Job drawing, mm, ordinate dimensions from the low corner. One solid piece. A direction names the side the tool comes from. Give positions to 0.01 mm unless a question says otherwise; leave off trailing zeros. Order: outer loops, then holes, each group sorted by start corner. A loop starts at its lowest first (then second) coordinate and runs counter-clockwise, first axis right, second up.
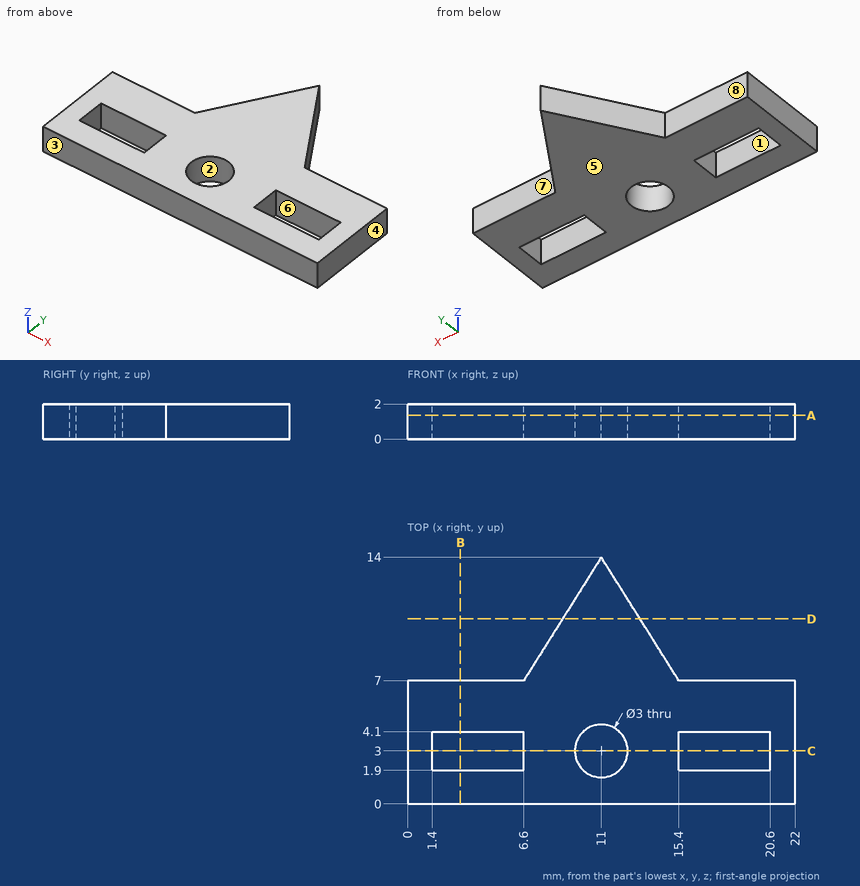
Item 1: Drill centre lines: probe 1 along X at (y, z) = (3.5, 1.85); probe 2 along Y at (x, z) = (16, 0.75); probe 3 along X at (y, z) = (2.75, 0.3). Where is each one in solid material? Low to high.
Item 2: Which spindle directions (+Z, -Z, +X, -X, +Y, -Y) get a long thin tool onto all of the face, cutting with end or side? Do the marked faces 5, 6, 7 and 8. Say none if no direction does.
Item 3: Band-saw the part on C-C on y = 3. List the corners of the cut face in (x, z), plus the area to 3 significant figures.
Item 4: Band-saw the part on D-D on y = 10.5. List the corners of the cut face in (x, z), plus the area to 3 significant figures.
Item 5: Band-saw the part on B-B on x = 3. List the corners of the cut face in (y, z), plus the area to 3 significant figures.
Item 6: Drop a flat-ended pin along its axis: P1, Ø0.6, axis at x = 2.5, z = 0.5, coming from the +Y side. Give the stop position or say it passes through.
Item 7: Band-saw the part on A-A on z = 1.35. List the corners of the cut face in (x, y).
Item 8: Pull direction Y, two halves, no side cores. Call the marked faces 1, 2, 3 and 4: released by +Y, released by -Y, zero draft, split by the parting line, or undercut.
Working result:
1. probe 1: x = 0 to 1.4, 6.6 to 9.59, 12.41 to 15.4, 20.6 to 22
1. probe 2: y = 0 to 1.9, 4.1 to 7
1. probe 3: x = 0 to 1.4, 6.6 to 9.52, 12.48 to 15.4, 20.6 to 22
2. face 5: -Z, +X, -X, +Y, -Y
2. face 6: +Z, -Z
2. face 7: +Z, -Z, +X, +Y
2. face 8: +Z, -Z, -X, +Y
3. outline: (0, 0) - (1.4, 0) - (1.4, 2) - (0, 2) - close; (6.6, 0) - (9.5, 0) - (9.5, 2) - (6.6, 2) - close; (12.5, 0) - (15.4, 0) - (15.4, 2) - (12.5, 2) - close; (20.6, 0) - (22, 0) - (22, 2) - (20.6, 2) - close
3. area: 17.2 mm2
4. outline: (8.8, 0) - (13.2, 0) - (13.2, 2) - (8.8, 2) - close
4. area: 8.80 mm2
5. outline: (0, 0) - (1.9, 0) - (1.9, 2) - (0, 2) - close; (4.1, 0) - (7, 0) - (7, 2) - (4.1, 2) - close
5. area: 9.60 mm2
6. P1: stops at y = 7
7. outline: (0, 0) - (22, 0) - (22, 7) - (15.4, 7) - (11, 14) - (6.6, 7) - (0, 7) - close; hole (1.4, 1.9) - (6.6, 1.9) - (6.6, 4.1) - (1.4, 4.1) - close; hole circle Ø3 at (11, 3); hole (15.4, 1.9) - (20.6, 1.9) - (20.6, 4.1) - (15.4, 4.1) - close
8. face 1: undercut
8. face 2: undercut
8. face 3: released by -Y
8. face 4: zero draft
